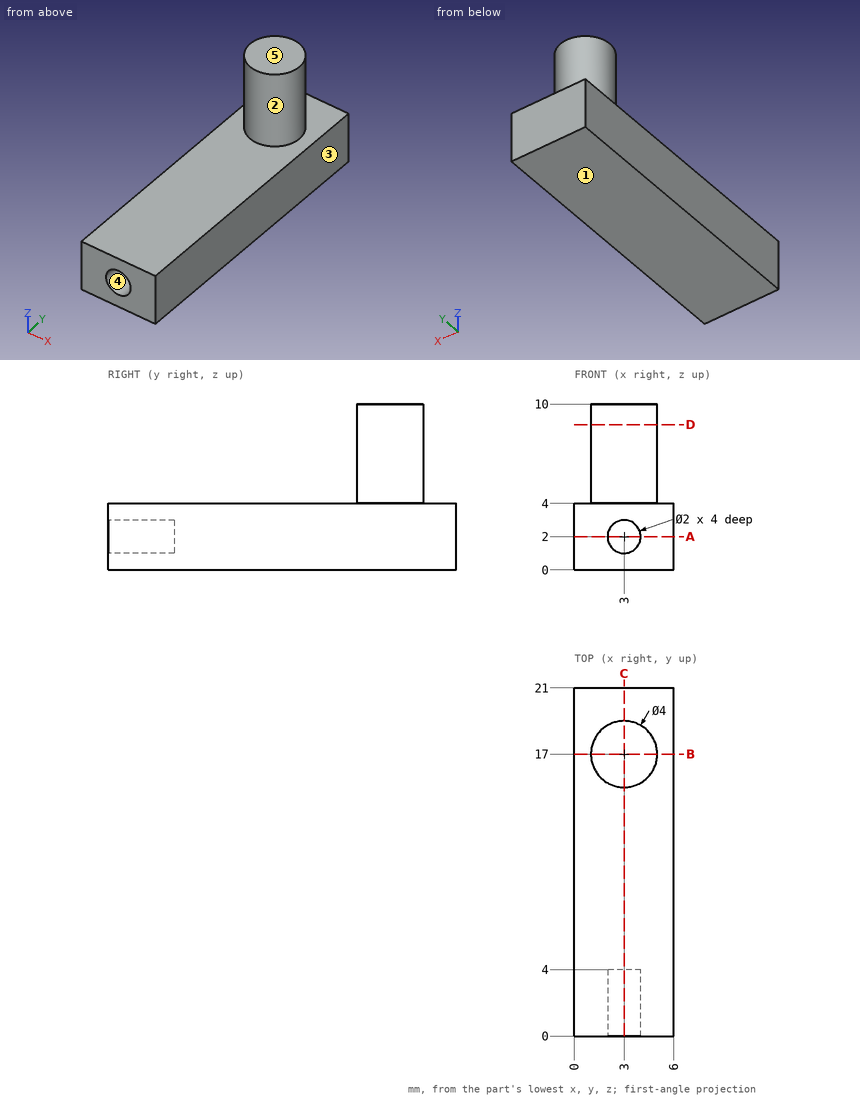
Check sheet for the drawn part. Datum: minimum x, y, z corner. Units: mm. A direction names the side the tool comes from. Coordinates: 2 decimals unless noted, no trailing zeros. Order: outer loops, then holes, each group sorted by start corner. A loop starts at its lowest first (then second) coordinate and runs counter-clockwise, first axis right, second up. Notation, with made-up numbers: (85.25, 4.25) -> (108.25, 4.25) arc R27 ccw to (108.25, 25.25) -> close; hole circle Ø4 at (87.5, -29). An arc over 180 degrees is marked (long way). Write each question's results on one line, items separated by ' | '. Start each with the question number.
1) Set-up check for the marked faces 1 and 2: record each of +Z, -Z, +X, -X, +Y, -Y from which the full face is reachable in a straight line by a thin tool's end or side.
2) Section check A-A (z = 2). Enter the section's corners in (x, y).
3) Draft check along X on the marked faces 3, 4 and 5. Enter one of: pulls with the +X half, pulls with the -X half, needs draft (parallel to the pull), parting line crosses it, or undercut.
4) Section check B-B (y = 17). Enter the section's corners in (x, z).
5) Section check D-D (z = 8.75). Enter the section's corners in (x, y).
6) Material ranges on line 1 along Z through (x, y) = (3, 3.05); line 2 along Z through (x, y) = (5.15, 8.5); line 3 along Y through (x, z) = (1.45, 8.5), recorded low to high.
7) Section check C-C (x = 3). Enter the section's corners in (y, z).
8) Depth check by flat-ended pin: pin 1 (1.2 mm diameter, centred on x = 3, z = 2, fed in from -Y); pin 2 (1.5 mm diameter, centred on x = 2, z = 8.5, fed in from -Y); pin 3 (1.5 mm diameter, centred on x = 1, y = 3.5, fed in from +Z). Enter the tip coordinate at first touch or a pass-through.
Checked values:
1) face 1: -Z, +X, -X, +Y, -Y | face 2: +Z
2) outline: (0, 0) -> (2, 0) -> (2, 4) -> (4, 4) -> (4, 0) -> (6, 0) -> (6, 21) -> (0, 21) -> close
3) face 3: pulls with the +X half | face 4: undercut | face 5: needs draft
4) outline: (0, 0) -> (6, 0) -> (6, 4) -> (5, 4) -> (5, 10) -> (1, 10) -> (1, 4) -> (0, 4) -> close
5) outline: circle Ø4 at (3, 17)
6) line 1: 0 to 1, 3 to 4 | line 2: 0 to 4 | line 3: 15.74 to 18.26
7) outline: (0, 0) -> (21, 0) -> (21, 4) -> (19, 4) -> (19, 10) -> (15, 10) -> (15, 4) -> (0, 4) -> (0, 3) -> (4, 3) -> (4, 1) -> (0, 1) -> close
8) pin 1: y = 4 | pin 2: y = 15.02 | pin 3: z = 4
